from build123d import *

# Parameters (mm, degrees)
CROQUIS1_W              = 426.64
CROQUIS1_H              = 400
SALIENTE_EXTRUIR1_DEPTH = 10
CROQUIS2_W              = 33.32
CROQUIS2_H              = 33.32
CORTAR_EXTRUIR1_DEPTH   = 393.634757764
CORTAR_EXTRUIR2_DEPTH   = 393.634757764


with BuildPart() as part:
    # Croquis1 → Saliente-Extruir1 (new body)
    with BuildSketch(Plane.XY):
        with Locations((80.724304492, -60)):
            Rectangle(CROQUIS1_W, CROQUIS1_H)
    extrude(amount=SALIENTE_EXTRUIR1_DEPTH)

    # Croquis2 → Cortar-Extruir1 (cut, through all)
    with BuildSketch(Plane.XY.offset(10)):
        with Locations((-115.935695508, -243.34)):
            Rectangle(CROQUIS2_W, CROQUIS2_H)
        with Locations((-115.935695508, 123.34)):
            Rectangle(CROQUIS2_W, CROQUIS2_H)
        with Locations((277.384304492, 123.34)):
            Rectangle(CROQUIS2_W, CROQUIS2_H)
        with Locations((277.384304492, -243.34)):
            Rectangle(CROQUIS2_W, CROQUIS2_H)
    extrude(amount=-CORTAR_EXTRUIR1_DEPTH, mode=Mode.SUBTRACT)

    # Croquis3 → Cortar-Extruir2 (cut, through all)
    with BuildSketch(Plane.XY.offset(10)):
        Polygon((-132.595695508, -137.05), (-132.595695508, -226.68), (-99.275695508, -226.68), (-99.275695508, -260), (-32.595695508, -260), (-32.595695508, -137.05), align=None)
    extrude(amount=-CORTAR_EXTRUIR2_DEPTH, mode=Mode.SUBTRACT)


solid = part.part
The listing builds one solid part. Answer for the finished solid, in the listing's coordinates (mm). A direction names the side the tool comes from. Give positions to 0.01 mm unless a question says otherwise; leave off trailing zeros. Order: outer loops, then holes, each group sorted by start corner. A loop starts at its lowest first (then second) coordinate and runs counter-clockwise, first axis right, second up. Notation, with made-up numbers: (30, -24.75) - (68, -24.75) arc R12 ccw to (68, -5.75) - close; hole circle Ø11 at (-33, -37). An arc over 180 degrees is marked (long way). Answer as CSV lines item,"result".
Q1. A cutting plane is placed at B-B, the plane y = -195. Determine the outline of the cut face in (x, z), and give its area (3 significant figures).
Answer key:
outline,"(-32.6, 0) - (294.04, 0) - (294.04, 10) - (-32.6, 10) - close"
area,"3,270 mm^2"
Q2. Each of these flat-tipped pins is pushed along its axis until it touches: pin 1 Ø3 at (x, z) = (270, 3.5) entering from -Y; pin 2 Ø3 at (x, z) = (273.5, 4.5) entering from +Y; pin 3 Ø5 at (y, z) = (131, 3) entering from +X. Where does it stop, or does it pass through?
Answer key:
pin 1,"stops at y = -226.68"
pin 2,"stops at y = 106.68"
pin 3,"stops at x = 260.72"
Q3. Which of the six approach directions +Z, -Z, +X, -X, +Y, -Y give full straight-line access (tool end or side, diameter ignored) to faces 1 (the face through (-32.596, -199, 5)), 2 (the face through (260.724, 123, 5)), 3 (the face through (277, -226.68, 5))?
Answer key:
face 1,"+Z, -Z, -X, -Y"
face 2,"+Z, -Z, +X, +Y"
face 3,"+Z, -Z, +X, -Y"
Q4. A cutting plane is placed at A-A, the plane z = 5.25. Determine the outline of the cut face in (x, y).
Answer key:
outline,"(-132.6, -137.05) - (-32.6, -137.05) - (-32.6, -260) - (260.72, -260) - (260.72, -226.68) - (294.04, -226.68) - (294.04, 106.68) - (260.72, 106.68) - (260.72, 140) - (-99.28, 140) - (-99.28, 106.68) - (-132.6, 106.68) - close"
Q5. Straight lines are drawn through the part: L1, parallel to X at y = -236, z = 5.5; L2, parallel to X at y = 116, z = 4; L3, parallel to Y at x = -55.5, z = 5. For each, find the intervals that lie inside material, in ascending order.
Answer key:
L1,"x = -32.6 to 260.72"
L2,"x = -99.28 to 260.72"
L3,"y = -137.05 to 140"
